Geometry check sheet. Reference: the model listing, model coordinates, mm. A direction names the side the tool comes from. Give positions to 0.01 mm unless a question says otherwise; leave off trailing zeros. Write each loop counter-clockwise with the first axis right and the second up, starting at its lowest first coordinate (ties: lowest second). Pieces come first, ordered by that corner, then holes. Notation, with made-up numbers: M 45,-23.5 L 87,-23.5 A20 cw 87,5.5 Z; hole C 39,37 d8. An arc over 180 degrees is marked long. One line per item, written item: value. Start each with the question number.
1. Cross-section at D-D on x = -25. Record the cut outline in (y, z).
2. Gauge pin test, flat end, axial feed: pin 1 (7 mm diameter, centred on x = -25, y = -25, fed in from +Z). Record the tip position at first contact, or that the pin passes through.
3. Cross-section at B-B on z = 0.5. Count the separate pieces of the cut face and the enclosed holes in it, then the cut area to 3 significant figures.
4. Cross-section at A-A on y = 25. Record the cut outline in (x, z), then the cut area to 3 significant figures.
5. Tool access check on faces 4 (the face through (1, -16, 1)), 5 (the face through (30, 0, 1)). Record the directions out of +Z, -Z, +X, -X, +Y, -Y that give a thin tool (end or side, any length) a straight path to the whole face; none if there is none.
6. Scan lines: line 1 (X direction, y = -9, z = 0.6); line 2 (Y direction, x = -10, z = 0.6); line 3 (Y direction, x = 25, z = 0.8). Record each from-to range of solid material in increasing order.
7. Cross-section at C-C on y = 4. Record the cut outline in (x, z), then the cut area to 3 significant figures.
8. Release check for a two-part mould opening along Y. For faces 1 (the face through (-1, 16, 1)), 2 (the face through (0, 0, 0)), 3 (the face through (28.859, -28.797, 0.74)) record: pulls with the +Y half, pulls with the -Y half, needs draft (parallel to the pull), parting line crosses it, or undercut.
Autodesk Inventor part; units mm, degrees
ref_plane "YZ Plane" through (0, 0, 0) normal (1, 0, 0) x (0, 1, 0)
ref_plane "XZ Plane" through (0, 0, 0) normal (0, 1, 0) x (-1, 0, 0)
ref_plane "XY Plane" through (0, 0, 0) normal (0, 0, 1) x (1, 0, 0)
sketch "Sketch1" plane through (0, 0, 0) normal (0, 0, 1) x (1, 0, 0)
  line L0 (-20, 30) -> (20, 30)
  line L1 (20, 30) -> (20, -30)
  line L2 (20, -30) -> (-20, -30)
  line L3 (-20, -30) -> (-20, 30)
  line L4 (-20, 30) -> (-26, 30)
  line L5 (-30, 26) -> (-30, -26)
  line L6 (-26, -30) -> (-20, -30)
  line L7 (-20, -30) -> (-20, 30)
  line L8 (20, 30) -> (26, 30)
  line L9 (30, 26) -> (30, -26)
  line L10 (26, -30) -> (20, -30)
  line L11 (20, -30) -> (20, 30)
  line L12 (-43.9092, 0) -> (47.176, 0) construction
  circle A0 centre (-25, 0) radius 2.25
  line L13 (-30, 20) -> (30, 20) construction
  circle A1 centre (-25, 25) radius 2.25
  line L14 (-30, -20) -> (30, -20) construction
  circle A2 centre (-25, -25) radius 2.25
  line L15 (-30, 5) -> (30, 5) construction
  line L16 (-30, -5) -> (30, -5) construction
  line L17 (-28, 18) -> (-22, 18)
  line L18 (-22, 18) -> (-22, 7)
  line L19 (-22, 7) -> (-28, 7)
  line L20 (-28, 7) -> (-28, 18)
  line L21 (-18, 28) -> (18, 28)
  line L22 (18, 28) -> (18, -28)
  line L23 (18, -28) -> (-18, -28)
  line L24 (-18, -28) -> (-18, 28)
  line L25 (-18, 1) -> (18, 1)
  line L26 (18, 1) -> (18, -1)
  line L27 (18, -1) -> (-18, -1)
  line L28 (-18, -1) -> (-18, 1)
  line L29 (-1, 28) -> (1, 28)
  line L30 (1, 28) -> (1, -28)
  line L31 (1, -28) -> (-1, -28)
  line L32 (-1, -28) -> (-1, 28)
  arc A3 (-26, 30) -> (-30, 26) centre (-26, 26) ccw
  arc A4 (-30, -26) -> (-26, -30) centre (-26, -26) ccw
  arc A5 (26, -30) -> (30, -26) centre (26, -26) ccw
  arc A6 (30, 26) -> (26, 30) centre (26, 26) ccw
  circle A7 centre (0, 0) radius 5
  point P0 (0, 30)
  point P1 (20, 0)
  point P2 (-30, -30)
  point P3 (30, -30)
  point P4 (-18, 0)
  point P5 (0, 28)
  dimension "d0" = 40
  dimension "d1" = 60
  dimension "d2" = 10
  dimension "d3" = 10
  dimension "d4" = 4.5
  dimension "d5" = 10
  dimension "d6" = 4.5
  dimension "d7" = 5
  dimension "d8" = 4.5
  dimension "d9" = 5
  dimension "d10" = 5
  dimension "d11" = 5
  dimension "d12" = 5
  dimension "d13" = 10
  dimension "d14" = 5
  dimension "d15" = 5
  dimension "d16" = 2
  dimension "d17" = 2
  dimension "d18" = 2
  dimension "d19" = 2
  dimension "d20" = 2
  dimension "d21" = 2
  dimension "d22" = 2
  dimension "d23" = 2
  dimension "d24" = 2
  dimension "d25" = 2
  dimension "d26" = 4
  dimension "d33" = 10
extrude "Extrusion1" add sketch "Sketch1" along normal blind 1.5 contours L0 L1 L2 L3 | L3 L6 A4 L5 A3 L4 | L8 A6 L9 A5 L10 L1 | A0 | A1 | A2 | L17 L18 L19 L20 | L21 L30 A7 L32 | L25 A7 L27 L24 | A7 L30 L25 L32 | L32 L25 A7 | L25 L32 L27 A7 | A7 L25 L30 | L25 L30 L27 L32 | L27 L32 A7 | L22 L27 A7 L25 | L25 A7 L27 L30 | L27 L30 A7 L32 | L32 A7 L30 L23 | L27 A7 L30
extrude "Extrusion2" cut sketch "Sketch1" along normal blind 2 contours A0 | A1 | A2
mirror "Mirror2" about plane through (0, 0, 0) normal (1, 0, 0) of "Extrusion2"
equation "\"d4\" = screw"
equation "\"d6\" = screw"
equation "\"d8\" = screw"
equation "\"screw\" = 4.5"
properties part number "MechBottomPlate"
Report:
1. outline: M -30,0 L -27.25,0 L -27.25,1.5 L -30,1.5 Z; M -22.75,0 L -2.25,0 L -2.25,1.5 L -22.75,1.5 Z; M 2.25,0 L 22.75,0 L 22.75,1.5 L 2.25,1.5 Z; M 27.25,0 L 30,0 L 30,1.5 L 27.25,1.5 Z
2. pin 1: stops at z = 1.5
3. separate pieces: 1
3. enclosed holes: 10
3. area: 1,700 mm^2
4. outline: M -30,0 L -27.25,0 L -27.25,1.5 L -30,1.5 Z; M -22.75,0 L -18,0 L -18,1.5 L -22.75,1.5 Z; M -1,0 L 1,0 L 1,1.5 L -1,1.5 Z; M 18,0 L 22.75,0 L 22.75,1.5 L 18,1.5 Z; M 27.25,0 L 30,0 L 30,1.5 L 27.25,1.5 Z
4. area: 25.5 mm^2
5. face 4: +Z, -Z
5. face 5: +Z, -Z, +X, +Y, -Y
6. line 1: x = -30 to -18, -1 to 1, 18 to 30
6. line 2: y = -30 to -28, -1 to 1, 28 to 30
6. line 3: y = -30 to -27.25, -22.75 to -2.25, 2.25 to 22.75, 27.25 to 30
7. outline: M -30,0 L -18,0 L -18,1.5 L -30,1.5 Z; M -3,0 L 3,0 L 3,1.5 L -3,1.5 Z; M 18,0 L 30,0 L 30,1.5 L 18,1.5 Z
7. area: 45.0 mm^2
8. face 1: undercut
8. face 2: needs draft
8. face 3: pulls with the -Y half
